Source: CAD feature listing. Evaluate the final solid. Frame: model axes, mm. Face numbers are marked on the shaded views. A direction names the side the tool comes from. Round coordinates to 2 decimals unless told otherwise and drop trailing zeros. Loops run counter-clockwise (first coordinate to the right, second up) from the corner with the lowest first, then second, coordinate; pieces in that order, holes last. Notation, with made-up numbers: (-17, 46) - (31, 46) arc R27 cw to (31, 77) - close; hole circle Ø6 at (-15.5, 78). An arc over 180 degrees is marked (long way). One line per question, with ' | ' between items. Start each with the question number.
1. Access query for the marked faces 4, 5, 6, 7 and 8. Directions: +Z, -Z, +X, -X, +Y, -Y. A direction counts if a zero-diameter tool reaches every point of the face in a straight line with its end or side. Return the directions, or none.
2. Cut plane D-D (y = 2). Return loops of the section in (x, z).
3. Pin query (flat end, axial travel): pin 1 (2.5 mm diameter, centred on x = 1, y = 15, fed in from +Z); pin 2 (12 mm diameter, centred on y = 9, z = -10.5, fed in from +X); pin 3 (3 mm diameter, centred on x = 3.5, z = 4.5, fed in from -Y); pin 4 (4 mm diameter, centred on x = 0, y = 20, fed in from -Z). Return the tip coordinate at first contact, or that it passes through.
4. Cut plane C-C (x = 0). Return loops of the section in (y, z), then the cut area to 3 significant figures.
5. Mould query, pull axis X, two halves, no side actions, for the marked faces 1, 2 and 3. Classes: pulls with the +X half, pulls with the -X half, needs draft (parallel to the pull), parting line crosses it, or undercut.
6. Ray query, line 1 (Z direction, x = -11.5, y = 7.5); line 2 (Y direction, x = 0, z = -7); line 3 (X direction, y = 23, z = 0). Return the intervals inside material, ascending.
7. Cut plane B-B (y = 14). Return loops of the section in (x, z).
8. Cut plane A-A (z = 0). Return loops of the section in (x, y), then the cut area to 3 significant figures.
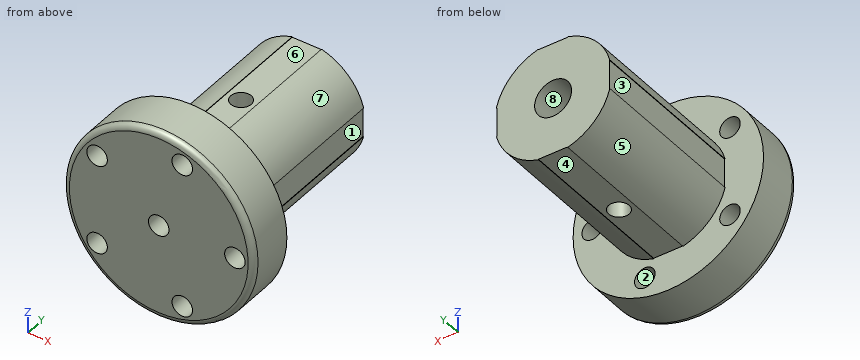
```python
from build123d import *

# Parameters (mm, degrees)
SKETCH1_R           = 16.25
BOSS_EXTRUDE1_DEPTH = 8
SKETCH2_R           = 10
BOSS_EXTRUDE2_DEPTH = 28
SKETCH3_R           = 3.15
CUT_EXTRUDE1_DEPTH  = 25
SKETCH4_W           = 1.193492023
SKETCH4_H           = 5
CUT_EXTRUDE2_DEPTH  = 28
CIRPATTERN1_COUNT   = 4
SKETCH5_R           = 1.75
CUT_EXTRUDE3_DEPTH  = 25
FILLET1_R           = 1
SKETCH6_R           = 1.75
CUT_EXTRUDE4_DEPTH  = 25
SKETCH7_R           = 1.75
CUT_EXTRUDE5_DEPTH  = 10
CIRPATTERN2_COUNT   = 5


with BuildPart() as part:
    # Sketch1 → Boss-Extrude1 (new body)
    with BuildSketch(Plane(origin=(0, 0, 0), x_dir=(1, 0, 0), z_dir=(0, 1, 0))):
        with Locations(Location((0, 0, 0), (0, 0, 270))):
            Circle(SKETCH1_R)
    extrude(amount=BOSS_EXTRUDE1_DEPTH)

    # Sketch2 → Boss-Extrude2 (add)
    with BuildSketch(Plane(origin=(0, 8, 0), x_dir=(1, 0, 0), z_dir=(0, 1, 0))):
        with Locations(Location((0, 0, 0), (0, 0, 270))):
            Circle(SKETCH2_R)
    extrude(amount=BOSS_EXTRUDE2_DEPTH)

    # Sketch3 → Cut-Extrude1 (cut)
    with BuildSketch(Plane(origin=(0, 36, 0), x_dir=(1, 0, 0), z_dir=(0, 1, 0))):
        with Locations(Location((0, 0, 0), (0, 0, 270))):
            Circle(SKETCH3_R)
    extrude(amount=-CUT_EXTRUDE1_DEPTH, mode=Mode.SUBTRACT)

    # Sketch4 → Cut-Extrude2 (cut)
    with BuildSketch(Plane(origin=(0, 36, 0), x_dir=(1, 0, 0), z_dir=(0, 1, 0))):
        with Locations((10.196746012, 0)):
            Rectangle(SKETCH4_W, SKETCH4_H)
    cut_extrude2 = extrude(amount=-CUT_EXTRUDE2_DEPTH, mode=Mode.SUBTRACT)

    # CirPattern1: Cut-Extrude2 ×4 about axis
    cirpattern1_axis = Axis((0, 0, 0), (0, 1, 0))
    for i in range(1, CIRPATTERN1_COUNT):
        add(cut_extrude2.rotate(cirpattern1_axis, i * 360 / CIRPATTERN1_COUNT), mode=Mode.SUBTRACT)

    # Sketch5 → Cut-Extrude3 (cut)
    with BuildSketch(Plane(origin=(0, 0, -9.6), x_dir=(-1, 0, 0), z_dir=(0, 0, -1))):
        with Locations((0, 20)):
            Circle(SKETCH5_R)
    extrude(amount=-CUT_EXTRUDE3_DEPTH, mode=Mode.SUBTRACT)

    # Fillet1
    fillet1_edges = [part.edges().sort_by_distance(p)[0] for p in [
        (0, 0, -16.25),
    ]]
    fillet(fillet1_edges, radius=FILLET1_R)

    # Sketch6 → Cut-Extrude4 (cut)
    with BuildSketch(Plane(origin=(0, 0, 0), x_dir=(-1, 0, 0), z_dir=(0, -1, 0))):
        with Locations(Location((0, 0, 0), (0, 0, 90))):
            Circle(SKETCH6_R)
    extrude(amount=-CUT_EXTRUDE4_DEPTH, mode=Mode.SUBTRACT)

    # Sketch7 → Cut-Extrude5 (cut)
    with BuildSketch(Plane(origin=(0, 0, 0), x_dir=(-1, 0, 0), z_dir=(0, -1, 0))):
        with Locations(Location((-13, 0, 0), (0, 0, 90))):
            Circle(SKETCH7_R)
    cut_extrude5 = extrude(amount=-CUT_EXTRUDE5_DEPTH, mode=Mode.SUBTRACT)

    # CirPattern2: Cut-Extrude5 ×5 about axis
    cirpattern2_axis = Axis((0, 0, 0), (0, 1, 0))
    for i in range(1, CIRPATTERN2_COUNT):
        add(cut_extrude5.rotate(cirpattern2_axis, i * 360 / CIRPATTERN2_COUNT), mode=Mode.SUBTRACT)


solid = part.part
```
Answers follow:
1) face 4: -Z, +Y | face 5: -Z, -X, +Y | face 6: +Z, +Y | face 7: +Z, +X, +Y | face 8: +Y
2) outline: circle Ø32.5 at (0, 0); hole circle Ø3.5 at (-10.52, -7.64); hole circle Ø3.5 at (-10.52, 7.64); hole circle Ø3.5 at (0, 0); hole circle Ø3.5 at (4.02, -12.36); hole circle Ø3.5 at (4.02, 12.36); hole circle Ø3.5 at (13, 0)
3) pin 1: stops at z = 9.6 | pin 2: stops at x = 15.59 | pin 3: stops at y = 0 | pin 4: stops at z = -9.6
4) outline: (0, -15.25) arc R1 ccw to (1, -16.25) - (8, -16.25) - (8, -9.6) - (18.25, -9.6) - (18.25, -3.15) - (11, -3.15) - (11, -1.75) - (0, -1.75) - close; (0, 1.75) - (11, 1.75) - (11, 3.15) - (18.25, 3.15) - (18.25, 9.6) - (8, 9.6) - (8, 16.25) - (1, 16.25) arc R1 ccw to (0, 15.25) - close; (21.75, -9.6) - (36, -9.6) - (36, -3.15) - (21.75, -3.15) - close; (21.75, 3.15) - (36, 3.15) - (36, 9.6) - (21.75, 9.6) - close | area: 556 mm2
5) face 1: pulls with the +X half | face 2: undercut | face 3: pulls with the -X half
6) line 1: z = -11.48 to -9.09, -6.19 to 6.19, 9.09 to 11.48 | line 2: y = 0 to 18.25, 21.75 to 36 | line 3: x = -9.6 to -3.15, 3.15 to 9.6
7) outline: (-9.68, -2.5) arc R10 ccw to (-2.5, -9.68) - (-2.5, -9.6) - (2.5, -9.6) - (2.5, -9.68) arc R10 ccw to (9.68, -2.5) - (9.6, -2.5) - (9.6, 2.5) - (9.68, 2.5) arc R10 ccw to (2.5, 9.68) - (2.5, 9.6) - (-2.5, 9.6) - (-2.5, 9.68) arc R10 ccw to (-9.68, 2.5) - (-9.6, 2.5) - (-9.6, -2.5) - close; hole circle Ø6.3 at (0, 0)
8) outline: (-16.25, 1) arc R1 ccw to (-15.25, 0) - (-1.75, 0) - (-1.75, 11) - (-3.15, 11) - (-3.15, 36) - (-9.6, 36) - (-9.6, 8) - (-16.25, 8) - close; (1.75, 0) - (11.25, 0) - (11.25, 8) - (9.6, 8) - (9.6, 36) - (3.15, 36) - (3.15, 11) - (1.75, 11) - close; (14.75, 0) - (15.25, 0) arc R1 ccw to (16.25, 1) - (16.25, 8) - (14.75, 8) - close | area: 573 mm2
